Design review of the part built by this model. Coordinates are the model's own, in mm. Give positions to 0.01 mm unless a question says otherwise; leave off trailing zeros. Loops run counter-clockwise (first coordinate to the right, second up) from the corner with the lowest first, then second, coordinate; pieces in that order, holes last. Notation, with made-up numbers: M 43,68.5 L 55,68.5 A14 ccw 55,79.5 Z; hole C 40.25,-18.75 d7. An arc over 180 degrees is marked long. Answer as CSV lines item,"result".
```python
from build123d import *

# Parameters (mm, degrees)
SKETCH1_R           = 2.5
SKETCH1_R_2         = 1.6
SKETCH1_R_3         = 12.25
BOSS_EXTRUDE1_DEPTH = 2.5


with BuildPart() as part:
    # Sketch1 → Boss-Extrude1 (new body)
    with BuildSketch(Plane.XY.offset(1.25)):
        with BuildLine():
            Line((-21, 19), (-21, -37))
            ThreePointArc((-21, -37), (-20.414213562, -38.414213562), (-19, -39))
            Line((-19, -39), (19, -39))
            ThreePointArc((19, -39), (20.414213562, -38.414213562), (21, -37))
            Line((21, -37), (21, 19))
            ThreePointArc((21, 19), (20.414213562, 20.414213562), (19, 21))
            Line((19, 21), (-19, 21))
            ThreePointArc((-19, 21), (-20.414213562, 20.414213562), (-21, 19))
        make_face()
        with Locations((-12.5, -31)):
            Circle(SKETCH1_R, mode=Mode.SUBTRACT)
        with Locations((-15.5, 15.5)):
            Circle(SKETCH1_R_2, mode=Mode.SUBTRACT)
        with Locations((15.5, -15.5)):
            Circle(SKETCH1_R_2, mode=Mode.SUBTRACT)
        Circle(SKETCH1_R_3, mode=Mode.SUBTRACT)
        with Locations((-15.5, -15.5)):
            Circle(SKETCH1_R_2, mode=Mode.SUBTRACT)
        with Locations((15.5, 15.5)):
            Circle(SKETCH1_R_2, mode=Mode.SUBTRACT)
        with Locations((12.5, -31)):
            Circle(SKETCH1_R, mode=Mode.SUBTRACT)
    extrude(amount=-BOSS_EXTRUDE1_DEPTH)


solid = part.part
```
1. To check wall thickness, follow L1, parallel to Y at x = -12.5, z = 0; L2, parallel to Y at x = -15.5, z = 0.7; L3, parallel to Y at x = -11, z = 0.3. State the ranges of each line that lie inside material, in increasing order. Write a range as [from, to].
Answer block:
L1,"[-39, -33.5], [-28.5, 21]"
L2,"[-39, -17.1], [-13.9, 13.9], [17.1, 21]"
L3,"[-39, -33], [-29, -5.39], [5.39, 21]"
2. We need section A-A, the plane y = 0. Write out the cut boundary in (x, z), plus the area to 4 significant figures.
Answer block:
outline,"M -21,-1.25 L -12.25,-1.25 L -12.25,1.25 L -21,1.25 Z; M 12.25,-1.25 L 21,-1.25 L 21,1.25 L 12.25,1.25 Z"
area,"43.75 mm²"
3. We need section D-D, the plane y = -31. Write out the cut boundary in (x, z), plus the area to 3 significant figures.
Answer block:
outline,"M -21,-1.25 L -15,-1.25 L -15,1.25 L -21,1.25 Z; M -10,-1.25 L 10,-1.25 L 10,1.25 L -10,1.25 Z; M 15,-1.25 L 21,-1.25 L 21,1.25 L 15,1.25 Z"
area,"80.0 mm²"
4. We need section C-C, the plane x = 6.5. Write out the cut boundary in (y, z).
Answer block:
outline,"M -39,-1.25 L -10.38,-1.25 L -10.38,1.25 L -39,1.25 Z; M 10.38,-1.25 L 21,-1.25 L 21,1.25 L 10.38,1.25 Z"
5. The part is to be moulded in two halves that separate along Y. For faces 1 (the cylindrical face through (-20.43, -38.4, 0.02)), 2 (the flat face through (21, -9, 0)), 3 (the cylindrical face through (13.9, -15.43, 0.02)), say which applies: pulls with the +Y half, pulls with the -Y half, needs draft (parallel to the pull), parting line crosses it, or undercut.
Answer block:
face 1,"pulls with the -Y half"
face 2,"needs draft"
face 3,"undercut"
6. We need section B-B, the plane z = 0.4. Write out the cut boundary in (x, y).
Answer block:
outline,"M -21,-37 A2 ccw -19,-39 L 19,-39 A2 ccw 21,-37 L 21,19 A2 ccw 19,21 L -19,21 A2 ccw -21,19 Z; hole C -15.5,-15.5 d3.2; hole C -15.5,15.5 d3.2; hole C -12.5,-31 d5; hole C 0,0 d24.5; hole C 12.5,-31 d5; hole C 15.5,-15.5 d3.2; hole C 15.5,15.5 d3.2"
